The model under review builds one solid part; all positions refer to its coordinate system, in mm. A direction names the side the tool comes from. Give positions to 0.01 mm unless a question says otherwise; leave off trailing zeros. Order: outer loops, then holes, each group sorted by start corner. A loop starts at its lowest first (then second) coordinate and runs counter-clockwise, first axis right, second up. Notation, with made-up numbers: (82.5, 53.25) - (90.5, 53.25) arc R26 ccw to (90.5, 72.25) - close; hole circle Ø6 at (-30.5, 67). An arc over 180 degrees is marked (long way). Write item = value, one per line. Start each with the question number.
1. We need section A-A, the plane z = -5. Give the boundary of the cut face in (x, y).
2. Wall thickness on probe 1 along Y at (x, z) = (0, 2.25); probe 2 along Z at (x, y) = (-1, -5); probe 3 along Y at (x, z) = (-2, -6): over which ranges is each line inside the solid? List them lowest first.
3. We need section D-D, the plane y = 2. Give the boundary of the cut face in (x, z).
4. We need section B-B, the plane x = 0. Give the boundary of the cut face in (y, z), and give its area (3 significant figures).
5. For P1, Ø1.6, axis at y = -8, z = 0.5, coming from the -X side; P2, Ø8, axis at y = 6, z = -5, coming from the -X side; P3, Ø3, axis at x = 0.5, y = -7.5, coming from the +Z side, all flat-tipped, find the tip position at first contact; note any pin that passes through.
6. We need section C-C, the plane y = -0.25. Give the boundary of the cut face in (x, z).
7. Mouldability with a two-part tool opening along Y and no side actions: class faces 4 (the flat face through (0, 10, 0)), 5 (the cylindrical face through (0, -1, -1)), 6 (the flat face through (0, -10, 0)), 7 (the flat face through (1, -1, 10)) as pulls with the +Y half, pulls with the -Y half, needs draft (parallel to the pull), parting line crosses it, or undercut.
8. Machinability: for faces 1 (the flat face through (2, 7, 0)), 2 (the flat face through (-2, -7, 0)), 3 (the flat face through (2, -7, 0)), which of the approach directions +Z, -Z, +X, -X, +Y, -Y give a long, thin tool a straight path to every point of the face, cutting with its end or side? Answer none if there is none.
from build123d import *

# Parameters (mm, degrees)
F0_R     = 1
F1_DEPTH = 11
F2_DEPTH = 1
F3_DEPTH = 10


with BuildPart() as f1:
    # F0 (on Top) → F1 (new body)
    with BuildSketch(Plane.XY):
        with BuildLine():
            Line((-2, 3.0532769282), (-2, 3.9752358421))
            ThreePointArc((-2, 3.9752358421), (-4.45, 0), (-2, -3.9752358421))
            Line((-2, -3.9752358421), (-2, -3.0532769282))
            ThreePointArc((-2, -3.0532769282), (-3.65, 0), (-2, 3.0532769282))
        make_face()
        with BuildLine():
            ThreePointArc((-2, -3.9752358421), (0, -4.45), (2, -3.9752358421))
            Line((2, -3.9752358421), (2, -3.0532769282))
            ThreePointArc((2, -3.0532769282), (0, -3.65), (-2, -3.0532769282))
            Line((-2, -3.0532769282), (-2, -3.9752358421))
        make_face()
        with BuildLine():
            ThreePointArc((2, -3.9752358421), (3.78830437, -2.3347912112), (4.45, 0))
            ThreePointArc((4.45, 0), (3.78830437, 2.3347912112), (2, 3.9752358421))
            Line((2, 3.9752358421), (2, 3.0532769282))
            ThreePointArc((2, 3.0532769282), (3.211113514, 1.7352953639), (3.65, 0))
            ThreePointArc((3.65, 0), (3.211113514, -1.7352953639), (2, -3.0532769282))
            Line((2, -3.0532769282), (2, -3.9752358421))
        make_face()
        with BuildLine():
            Line((2, 3.0532769282), (2, 3.9752358421))
            ThreePointArc((2, 3.9752358421), (0, 4.45), (-2, 3.9752358421))
            Line((-2, 3.9752358421), (-2, 3.0532769282))
            ThreePointArc((-2, 3.0532769282), (0, 3.65), (2, 3.0532769282))
        make_face()
        with BuildLine():
            Line((-2, -3.0532769282), (-2, 3.0532769282))
            ThreePointArc((-2, 3.0532769282), (-3.65, 0), (-2, -3.0532769282))
        make_face()
        with BuildLine():
            Line((2, -3.0532769282), (2, 3.0532769282))
            ThreePointArc((2, 3.0532769282), (0, 3.65), (-2, 3.0532769282))
            Line((-2, 3.0532769282), (-2, -3.0532769282))
            ThreePointArc((-2, -3.0532769282), (0, -3.65), (2, -3.0532769282))
        make_face()
        Circle(F0_R, mode=Mode.SUBTRACT)
        with BuildLine():
            ThreePointArc((3.65, 0), (3.211113514, 1.7352953639), (2, 3.0532769282))
            Line((2, 3.0532769282), (2, -3.0532769282))
            ThreePointArc((2, -3.0532769282), (3.211113514, -1.7352953639), (3.65, 0))
        make_face()
    extrude(amount=-F1_DEPTH)

    # F0 (on Top) → F2 (join, symmetric)
    with BuildSketch(Plane.XY):
        with BuildLine():
            ThreePointArc((-2, 3.9752358421), (0, 4.45), (2, 3.9752358421))
            Line((2, 3.9752358421), (2, 10))
            Line((2, 10), (-2, 10))
            Line((-2, 10), (-2, 3.9752358421))
        make_face()
        with BuildLine():
            Line((2, -10), (2, -3.9752358421))
            ThreePointArc((2, -3.9752358421), (0, -4.45), (-2, -3.9752358421))
            Line((-2, -3.9752358421), (-2, -10))
            Line((-2, -10), (2, -10))
        make_face()
        with BuildLine():
            Line((2, 3.0532769282), (2, 3.9752358421))
            ThreePointArc((2, 3.9752358421), (0, 4.45), (-2, 3.9752358421))
            Line((-2, 3.9752358421), (-2, 3.0532769282))
            ThreePointArc((-2, 3.0532769282), (0, 3.65), (2, 3.0532769282))
        make_face()
        with BuildLine():
            ThreePointArc((-2, -3.9752358421), (0, -4.45), (2, -3.9752358421))
            Line((2, -3.9752358421), (2, -3.0532769282))
            ThreePointArc((2, -3.0532769282), (0, -3.65), (-2, -3.0532769282))
            Line((-2, -3.0532769282), (-2, -3.9752358421))
        make_face()
        with BuildLine():
            Line((-2, 3.0532769282), (-2, 3.9752358421))
            ThreePointArc((-2, 3.9752358421), (-4.45, 0), (-2, -3.9752358421))
            Line((-2, -3.9752358421), (-2, -3.0532769282))
            ThreePointArc((-2, -3.0532769282), (-3.65, 0), (-2, 3.0532769282))
        make_face()
        with BuildLine():
            ThreePointArc((2, -3.9752358421), (3.78830437, -2.3347912112), (4.45, 0))
            ThreePointArc((4.45, 0), (3.78830437, 2.3347912112), (2, 3.9752358421))
            Line((2, 3.9752358421), (2, 3.0532769282))
            ThreePointArc((2, 3.0532769282), (3.211113514, 1.7352953639), (3.65, 0))
            ThreePointArc((3.65, 0), (3.211113514, -1.7352953639), (2, -3.0532769282))
            Line((2, -3.0532769282), (2, -3.9752358421))
        make_face()
    extrude(amount=F2_DEPTH, both=True)

    # F0 (on Top) → F3 (join)
    with BuildSketch(Plane.XY):
        with BuildLine():
            Line((-2, -3.0532769282), (-2, 3.0532769282))
            ThreePointArc((-2, 3.0532769282), (-3.65, 0), (-2, -3.0532769282))
        make_face()
        with BuildLine():
            Line((2, -3.0532769282), (2, 3.0532769282))
            ThreePointArc((2, 3.0532769282), (0, 3.65), (-2, 3.0532769282))
            Line((-2, 3.0532769282), (-2, -3.0532769282))
            ThreePointArc((-2, -3.0532769282), (0, -3.65), (2, -3.0532769282))
        make_face()
        Circle(F0_R, mode=Mode.SUBTRACT)
        with BuildLine():
            ThreePointArc((3.65, 0), (3.211113514, 1.7352953639), (2, 3.0532769282))
            Line((2, 3.0532769282), (2, -3.0532769282))
            ThreePointArc((2, -3.0532769282), (3.211113514, -1.7352953639), (3.65, 0))
        make_face()
    extrude(amount=F3_DEPTH)


solid = f1.part
Model answer:
q1.outline = circle Ø8.9 at (0, 0); hole circle Ø2 at (0, 0)
q2.probe_1 = -3.65 to -1, 1 to 3.65
q2.probe_2 = -1 to 1
q2.probe_3 = -3.98 to 3.98
q3.outline = (-3.98, -11) - (3.98, -11) - (3.98, 1) - (3.05, 1) - (3.05, 10) - (-3.05, 10) - (-3.05, 1) - (-3.98, 1) - close
q4.outline = (-10, -1) - (-4.45, -1) - (-4.45, -11) - (-1, -11) - (-1, 10) - (-3.65, 10) - (-3.65, 1) - (-10, 1) - close; (1, -11) - (4.45, -11) - (4.45, -1) - (10, -1) - (10, 1) - (3.65, 1) - (3.65, 10) - (1, 10) - close
q4.area = 153 mm2
q5.P1 = -2
q5.P2 = -3.98
q5.P3 = 1
q6.outline = (-4.44, -11) - (-0.97, -11) - (-0.97, 10) - (-3.64, 10) - (-3.64, 1) - (-4.44, 1) - close; (0.97, -11) - (4.44, -11) - (4.44, 1) - (3.64, 1) - (3.64, 10) - (0.97, 10) - close
q7.face_4 = pulls with the +Y half
q7.face_5 = undercut
q7.face_6 = pulls with the -Y half
q7.face_7 = needs draft
q8.face_1 = +Z, -Z, +X, +Y
q8.face_2 = +Z, -Z, -X, -Y
q8.face_3 = +Z, -Z, +X, -Y
